Verification items for the finished model (mm, model axes). Give positions to 0.01 mm unless a question says otherwise; leave off trailing zeros. Write each loop counter-clockwise with the first axis right and the second up, starting at its lowest first coordinate (ties: lowest second). Pieces come first, ordered by that corner, then holes.
from build123d import *

# Parameters (mm, degrees)
F0_W     = 144.6518152952
F0_H     = 137.2342258692
F2_DEPTH = 25.4
F1_R     = 25.39999


# Not quite as in the source:
# - a fillet or chamfer is up to 0.001 mm smaller than in the source, because OpenCascade refuses the exact size


with BuildPart() as f2:
    # F0 (on Front) → F2 (new body)
    with BuildSketch(Plane.XZ):
        with Locations((23.3432799578, -12.742228806)):
            Rectangle(F0_W, F0_H)
    extrude(amount=F2_DEPTH)

    # F1 (radius 25.4 in the source; OpenCascade refuses exactly that, so slightly less here)
    f1_edges = [f2.edges().sort_by_distance(p)[0] for p in [
        (-48.982628, -12.7, 55.874884),
        (23.34328, -25.4, 55.874884),
        (-48.982628, -25.4, -12.742229),
    ]]
    fillet(f1_edges, radius=F1_R)


solid = f2.part
Item 1: Sectioned sample at A-A on y = -6.75. Record the cut outline in (x, z), then the cut area to 3 significant figures.
Answer key:
outline: (-48.07, -81.36) - (95.67, -81.36) - (95.67, 54.96) - (-23.58, 54.96) arc R24.49 ccw to (-48.07, 30.47) - close
area: 19,500 mm2
Item 2: Scan lines: line 1 along Z through (x, y) = (-18.5, -0.75); line 2 along X through (y, z) = (-1.25, -9.5); line 3 along Y through (x, z) = (-33, -68). Record each from-to range of solid material in increasing order.
Answer key:
line 1: z = -81.36 to 55.86
line 2: x = -48.95 to 95.67
line 3: y = -23.59 to 0
Item 3: Depth check by flat-ended pin: pin 1 (5 mm diameter, centred on x = 22.5, y = -16, fed in from +Z); pin 2 (10 mm diameter, centred on x = -1.5, y = -7, fed in from +Z); pin 3 (3 mm diameter, centred on y = -20.5, z = 1, fed in from -X). Enter the tip coordinate at first touch or a pass-through.
Answer key:
pin 1: stops at z = 51.99
pin 2: stops at z = 55.8
pin 3: stops at x = -40.44
